from build123d import *

# Parameters (mm, degrees)
BOSS_EXTRUDE1_START    = -63.5
BOSS_EXTRUDE1_DEPTH    = 57.15
SKETCH4_R              = 3.81
CUT_EXTRUDE2_DEPTH     = 12.7
CONVERT_SOLID3_START   = -274.103914115
CONVERT_SOLID3_DEPTH   = 57.15
CONVERT_SOLID3_2_DEPTH = 57.15
SKETCH13_R             = 3.175
CUT_EXTRUDE3_DEPTH     = 5.842


# Read off the part's stored shape, not the designer's step: Convert-Solid3
with BuildPart() as part:
    # Sketch3 → Boss-Extrude1 (new body)
    with BuildSketch(Plane.ZY.offset(337.603914115).offset(BOSS_EXTRUDE1_START)):
        Polygon((5.267071178, 203.186586599), (83.097186599, 137.879365455), (5.267071178, 72.698998764), align=None)
        Polygon((78.154944449, 137.881730876), (8.442071178, 196.377777126), (8.442071178, 79.499308876), align=None, mode=Mode.SUBTRACT)
    extrude(amount=-BOSS_EXTRUDE1_DEPTH)

    # Sketch4 → Cut-Extrude2 (cut)
    with BuildSketch(Plane(origin=(0, 121.82830981, 102.226089829), x_dir=(1, 0, 0), z_dir=(0, 0.7660444431189748, 0.6427876096865434))):
        with Locations(Location((-266.483914115, 56.721009713, 0), (0, 0, 270))):
            Circle(SKETCH4_R)
        with Locations(Location((-224.573914115, 56.721009713, 0), (0, 0, 270))):
            Circle(SKETCH4_R)
    extrude(amount=-CUT_EXTRUDE2_DEPTH, mode=Mode.SUBTRACT)

    # Convert-Solid3 outline → Convert-Solid3 (cut)
    with BuildSketch(Plane.YZ.offset(CONVERT_SOLID3_START)):
        Polygon((72.698998764, 5.267071178), (81.863084577, 5.267071178), (81.863084577, 8.442071178), (79.499308876, 8.442071178), (81.016980609, 10.254282003), (78.582837061, 12.292803573), align=None)
        with BuildLine():
            ThreePointArc((195.068228967, 8.442071178), (192.743967654, 6.117809864), (189.568967654, 5.267071178))
            Line((189.568967654, 5.267071178), (203.186586599, 5.267071178))
            Line((203.186586599, 5.267071178), (194.433349867, 15.6987725))
            ThreePointArc((194.433349867, 15.6987725), (195.822496885, 12.719737106), (195.536015795, 9.445243268))
            Line((195.536015795, 9.445243268), (196.377777126, 8.442071178))
            Line((196.377777126, 8.442071178), (195.068228967, 8.442071178))
        make_face()
        with BuildLine():
            Line((137.879365455, 83.097186599), (133.015809203, 77.289745437))
            ThreePointArc((133.015809203, 77.289745437), (137.881057106, 79.562701571), (142.748478512, 77.29440362))
            Line((142.748478512, 77.29440362), (137.879365455, 83.097186599))
        make_face()
    extrude(amount=CONVERT_SOLID3_DEPTH, mode=Mode.SUBTRACT)

    # Convert-Solid3 2 outline → Convert-Solid3 2 (add)
    with BuildSketch(Plane.YZ.offset(CONVERT_SOLID3_START)):
        with BuildLine():
            ThreePointArc((192.001158761, 13.657921839), (192.446494877, 10.275258197), (189.568967654, 8.442071178))
            Line((189.568967654, 8.442071178), (195.068228967, 8.442071178))
            ThreePointArc((195.068228967, 8.442071178), (195.324022101, 8.933445216), (195.536015795, 9.445243268))
            Line((195.536015795, 9.445243268), (192.001158761, 13.657921839))
        make_face()
        with BuildLine():
            ThreePointArc((135.44995275, 75.251223868), (137.882576702, 76.387701935), (140.316287405, 75.253552959))
            Line((140.316287405, 75.253552959), (137.881730876, 78.154944449))
            Line((137.881730876, 78.154944449), (135.44995275, 75.251223868))
        make_face()
    extrude(amount=CONVERT_SOLID3_2_DEPTH)

    # Sketch13 → Cut-Extrude3 (cut)
    with BuildSketch(Plane(origin=(0, 0, 5.267071178), x_dir=(-1, 0, 0), z_dir=(0, 0, -1))):
        with Locations((229.4949236, 107.263084577)):
            Circle(SKETCH13_R)
        with Locations((261.2449236, 107.263084577)):
            Circle(SKETCH13_R)
        with Locations((245.3699236, 151.713084577)):
            Circle(SKETCH13_R)
    extrude(amount=-CUT_EXTRUDE3_DEPTH, mode=Mode.SUBTRACT)


solid = part.part
The listing builds one solid part. Answer for the finished solid, in the listing's coordinates (mm). A direction names the side the tool comes from. Coordinates: 2 decimals unless noted, no trailing zeros. Loops run counter-clockwise (first coordinate to the right, second up) from the corner with the lowest first, then second, coordinate; pieces in that order, holes last.
1) Find section B-B on y = 114. Write down the section's boundary in (x, z), then the cut area to 3 significant figures.
2) Flat-ended cylindrical pins translate along their axes: pin 1 Ø5 at (x, y) = (-235.5, 105.5) entering from +Z; pin 2 Ø3 at (x, y) = (-265.5, 155.5) entering from +Z; pin 3 Ø8.5 at (x, y) = (-245.37, 151.71) entering from -Z; pin 4 Ø6 at (x, z) = (-238, 21) entering from -Y. Find the tip coordinate at first contact, or state that the pin passes through.
3) Find the intervals of material crossed by L1, parallel to Y at x = -266, z = 39; L2, parallel to Y at x = -266.5, z = 34; L3, parallel to Z at x = -232.5, y = 182, in increasing order.
4) A tool of negligible diameter and unlimited length cuts with its end or side. For faces 4 (the face through (-260.83, 110.41, 6.83)), 5 (the face through (-245.929, 165.797, 44.887)), 6 (the face through (-246, 136, 8.442)), 7 (the face through (-246, 81.863, 7)), 8 (the face through (-246, 135, 5.267)), from which of +Z, -Z, +X, -X, +Y, -Y can it reach the whole face along a straight path? Write none if from no direction.
5) Determine the mould class of faces 1 (the face through (-245.929, 137.844, 76.387)), 2 (the face through (-216.954, 137, 7)), 3 (the face through (-245.93, 168.95, 46.07)) for opening direction Y: pulls with the +Y half, pulls with the -Y half, needs draft (parallel to the pull), parting line crosses it, or undercut.
6) Find section A-A on x = -223. Write down the section's boundary in (y, z) (3 decimals).
7) Find section C-C on z = 30. Write down the section's boundary in (x, y).
Values:
1. outline: (-274.1, 5.27) - (-216.95, 5.27) - (-216.95, 8.44) - (-274.1, 8.44) - close; (-274.1, 49.64) - (-216.95, 49.64) - (-216.95, 54.58) - (-274.1, 54.58) - close
1. area: 464 mm2
2. pin 1: stops at z = 47.42
2. pin 2: stops at z = 63.89
2. pin 3: stops at z = 5.27
2. pin 4: stops at y = 83.36
3. L1: y = 100.95 to 105.09, 170.74 to 174.88
3. L2: y = 96.76 to 100.9, 174.93 to 179.08
3. L3: z = 5.27 to 8.44, 25.58 to 30.52
4. face 4: -Z
4. face 5: +X, -X
4. face 6: +X, -X, -Y
4. face 7: -Z, +X, -X, -Y
4. face 8: -Z, +X, -X, +Y, -Y
5. face 1: undercut
5. face 2: needs draft
5. face 3: pulls with the +Y half
6. outline: (78.583, 12.293) - (81.017, 10.254) - (135.45, 75.251) arc R3.175 cw to (140.316, 75.254) - (153.625, 59.392) - (156.058, 61.433) - (142.748, 77.294) arc R6.35 ccw to (133.016, 77.29) - close; (81.863, 5.267) - (189.569, 5.267) arc R6.35 ccw to (194.433, 15.699) - (160.518, 56.117) - (158.086, 54.076) - (192.001, 13.658) arc R3.175 cw to (189.569, 8.442) - (81.863, 8.442) - close
7. outline: (-274.1, 93.41) - (-216.95, 93.41) - (-216.95, 97.55) - (-274.1, 97.55) - close; (-274.1, 178.29) - (-216.95, 178.29) - (-216.95, 182.43) - (-274.1, 182.43) - close
